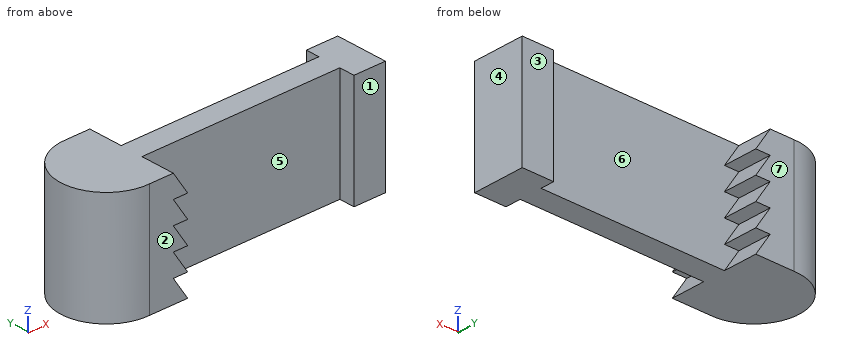
from build123d import *

# Parameters (mm, degrees)
F0_W     = 1.9128494449
F0_H     = 2
F1_DEPTH = 9.779
F3_DEPTH = 3
F5_DEPTH = 3


# Not quite as in the source:
# - a feature names something its author has since deleted; it is built from what else it names


with BuildPart() as f1:
    # F0 (on Top) → F1 (new body)
    with BuildSketch(Plane.XY):
        Polygon((14.9611846233, 0.28775621), (14.9611846233, -0.9137945543), (14.9611846233, -2.9137945543), (14.9611846233, -4.2726983058), (17.7320937316, -4.2726983058), (17.7320937316, 0.28775621), align=None)
        with BuildLine():
            Line((13.0483351785, -0.9137945543), (-0.8558859308, -0.9137945543))
            ThreePointArc((-0.8558859308, -0.9137945543), (-0.7608167592, -1.4097829714), (-0.7289579861, -1.9137945543))
            ThreePointArc((-0.7289579861, -1.9137945543), (-0.7608167592, -2.4178061373), (-0.8558859308, -2.9137945543))
            Line((-0.8558859308, -2.9137945543), (13.0483351785, -2.9137945543))
            Line((13.0483351785, -2.9137945543), (13.0483351785, -0.9137945543))
        make_face()
        with Locations((14.0047599009, -1.9137945543)):
            Rectangle(F0_W, F0_H)
        with BuildLine():
            Line((-4.7316648215, -2.9137945543), (-4.7316648215, -0.9137945543))
            Line((-4.7316648215, -0.9137945543), (-4.7316648215, 2.0862054457))
            Line((-4.7316648215, 2.0862054457), (-4.5844846254, 2.0862054457))
            ThreePointArc((-4.5844846254, 2.0862054457), (-8.7343716569, -1.9137945543), (-4.5844846254, -5.9137945543))
            Line((-4.5844846254, -5.9137945543), (-4.7316648215, -5.9137945543))
            Line((-4.7316648215, -5.9137945543), (-4.7316648215, -2.9137945543))
        make_face()
        with BuildLine():
            Line((-1.2312275376, -2.9137945543), (-4.7316648215, -2.9137945543))
            Line((-4.7316648215, -2.9137945543), (-4.7316648215, -5.9137945543))
            Line((-4.7316648215, -5.9137945543), (-4.5844846254, -5.9137945543))
            ThreePointArc((-4.5844846254, -5.9137945543), (-2.6374223247, -5.3249249204), (-1.2312275376, -3.8550830006))
            Line((-1.2312275376, -3.8550830006), (-1.2312275376, -2.9137945543))
        make_face()
        with BuildLine():
            Line((-4.7316648215, 2.0862054457), (-4.7316648215, -0.9137945543))
            Line((-4.7316648215, -0.9137945543), (-1.2264648215, -0.9137945543))
            Line((-1.2264648215, -0.9137945543), (-1.2264648215, 0.0188810444))
            ThreePointArc((-1.2264648215, 0.0188810444), (-2.6332302099, 1.4947585391), (-4.5844846254, 2.0862054457))
            Line((-4.5844846254, 2.0862054457), (-4.7316648215, 2.0862054457))
        make_face()
        with BuildLine():
            Line((-1.2264648215, -0.9137945543), (-4.7316648215, -0.9137945543))
            Line((-4.7316648215, -0.9137945543), (-4.7316648215, -2.9137945543))
            Line((-4.7316648215, -2.9137945543), (-1.2312275376, -2.9137945543))
            Line((-1.2312275376, -2.9137945543), (-0.8558859308, -2.9137945543))
            ThreePointArc((-0.8558859308, -2.9137945543), (-0.7608167592, -2.4178061373), (-0.7289579861, -1.9137945543))
            ThreePointArc((-0.7289579861, -1.9137945543), (-0.7608167592, -1.4097829714), (-0.8558859308, -0.9137945543))
            Line((-0.8558859308, -0.9137945543), (-1.2264648215, -0.9137945543))
        make_face()
        with BuildLine():
            Line((-1.2312275376, -5.9137945543), (-1.2312275376, -3.8550830006))
            ThreePointArc((-1.2312275376, -3.8550830006), (-2.6374223247, -5.3249249204), (-4.5844846254, -5.9137945543))
            Line((-4.5844846254, -5.9137945543), (-1.2312275376, -5.9137945543))
        make_face()
        with BuildLine():
            ThreePointArc((-4.5844846254, 2.0862054457), (-2.6332302099, 1.4947585391), (-1.2264648215, 0.0188810444))
            Line((-1.2264648215, 0.0188810444), (-1.2264648215, 2.0862054457))
            Line((-1.2264648215, 2.0862054457), (-4.5844846254, 2.0862054457))
        make_face()
    extrude(amount=F1_DEPTH)

    # F2 (on face) → F3 (cut)
    with BuildSketch(Plane.XZ.offset(5.9137945543)):
        Polygon((-1.2312275376, 0), (-1.2312275376, 1.9558), (-2.5021124942, 1.9558), align=None)
        Polygon((-1.2312275376, 1.9558), (-1.2312275376, 3.9116), (-2.5021124942, 3.9116), align=None)
        Polygon((-1.2312275376, 4.8895), (-1.2312275376, 5.8674), (-2.5021124942, 5.8674), (-1.2312275376, 3.9116), align=None)
        Polygon((-1.2312275376, 5.8674), (-1.2312275376, 7.8232), (-2.5021124942, 7.8232), align=None)
        Polygon((-1.2312275376, 9.779), (-2.5021124942, 9.779), (-1.2312275376, 7.8232), align=None)
    extrude(amount=-F3_DEPTH, mode=Mode.SUBTRACT)

    # F4 (on face) → F5 (cut)
    with BuildSketch(Plane(origin=(0, 2.0862054457, 0), x_dir=(-1, 0, 0), z_dir=(0, 1, 0))):
        Polygon((1.2264648215, 9.779), (1.2264648215, 7.8232), (2.4964648215, 9.779), align=None)
        Polygon((1.2264648215, 7.8232), (1.2264648215, 5.8674), (2.4964648215, 7.8232), align=None)
        Polygon((1.2264648215, 4.8895), (1.2264648215, 3.9116), (2.4964648215, 5.8674), (1.2264648215, 5.8674), align=None)
        Polygon((1.2264648215, 3.9116), (1.2264648215, 1.9558), (2.4964648215, 3.9116), align=None)
        Polygon((1.2264648215, 1.9558), (1.2264648215, 0), (2.4964648215, 1.9558), align=None)
    extrude(amount=-F5_DEPTH, mode=Mode.SUBTRACT)


solid = f1.part
Source: CAD feature listing. Evaluate the final solid. Frame: model axes, mm. Face numbers are marked on the shaded views. A direction names the side the tool comes from. Give positions to 0.01 mm unless a question says otherwise; leave off trailing zeros. Write each loop counter-clockwise with the first axis right and the second up, starting at its lowest first coordinate (ties: lowest second). Pieces come first, ordered by that corner, then holes. Notation, with made-up numbers: (-4.5, -34) - (52.5, -34) arc R14 ccw to (52.5, -17) - close; hole circle Ø4 at (-26.75, 7.5). An arc over 180 degrees is marked (long way). Write item = value, one per line. Start each with the question number.
Q1. Cut plane A-A, the plane y = -0.5. Return loops of the section in (x, z), then the cut area to 3 significant figures.
Q2. Cut plane C-C, the plane x = 12. Return loops of the section in (y, z), then the cut area to 3 significant figures.
Q3. Reachability of the marked faces 1, 2 and 3 from +Z, -Z, +X, -X, +Y, -Y: full face, straight path, thin tool, end or side. Return the list, or none.
Q4. Pin query (flat end, axial travel): pin 1 Ø4 at (x, z) = (1, 7.5) entering from -Y; pin 2 Ø1 at (x, y) = (14.5, -4) entering from +Z; pin 3 Ø1.4 at (x, z) = (16.5, 3) entering from -Y; pin 4 Ø1.7 at (x, z) = (-2, 3.5) entering from +Y. Return the tip coordinate at first contact, or that it passes through.
Q5. Material intervals for probe 1 along Y at (x, z) = (3, 1); probe 2 along X at (y, z) = (-0.75, 5.25); probe 3 along X at (y, z) = (-2.75, 0.75), sorted ascending.
Q6. Draft query along X for the marked faces 4, 5, 6 and 7. Return one class per face: +X half, -X half, draft (parallel to the pull), parting line (faces both ways), or undercut.
Q7. Cut plane D-D, the plane y = 1. Return loops of the section in (x, z).
Computed values:
q1.outline = (-8.48, 0) - (-1.23, 0) - (-2.5, 1.96) - (-1.23, 1.96) - (-2.5, 3.91) - (-1.23, 3.91) - (-2.5, 5.87) - (-1.23, 5.87) - (-2.5, 7.82) - (-1.23, 7.82) - (-2.5, 9.78) - (-8.48, 9.78) - close; (14.96, 0) - (17.73, 0) - (17.73, 9.78) - (14.96, 9.78) - close
q1.area = 91.8 mm²
q2.outline = (-2.91, 0) - (-0.91, 0) - (-0.91, 9.78) - (-2.91, 9.78) - close
q2.area = 19.6 mm²
q3.face_1 = +Z, -Z, +X, -Y
q3.face_2 = +Z, -Z, +X, -X, -Y
q3.face_3 = +Z, -Z, +X, +Y
q4.pin_1 = -2.91
q4.pin_2 = 9.78
q4.pin_3 = -4.27
q4.pin_4 = 2.09
q5.probe_1 = -2.91 to -0.91
q5.probe_2 = -8.56 to -2.1, 14.96 to 17.73
q5.probe_3 = -8.65 to 17.73
q6.face_4 = +X half
q6.face_5 = undercut
q6.face_6 = undercut
q6.face_7 = draft
q7.outline = (-7.48, 0) - (-1.23, 0) - (-2.5, 1.96) - (-1.23, 1.96) - (-2.5, 3.91) - (-1.23, 3.91) - (-2.5, 5.87) - (-1.23, 5.87) - (-2.5, 7.82) - (-1.23, 7.82) - (-2.5, 9.78) - (-7.48, 9.78) - close
